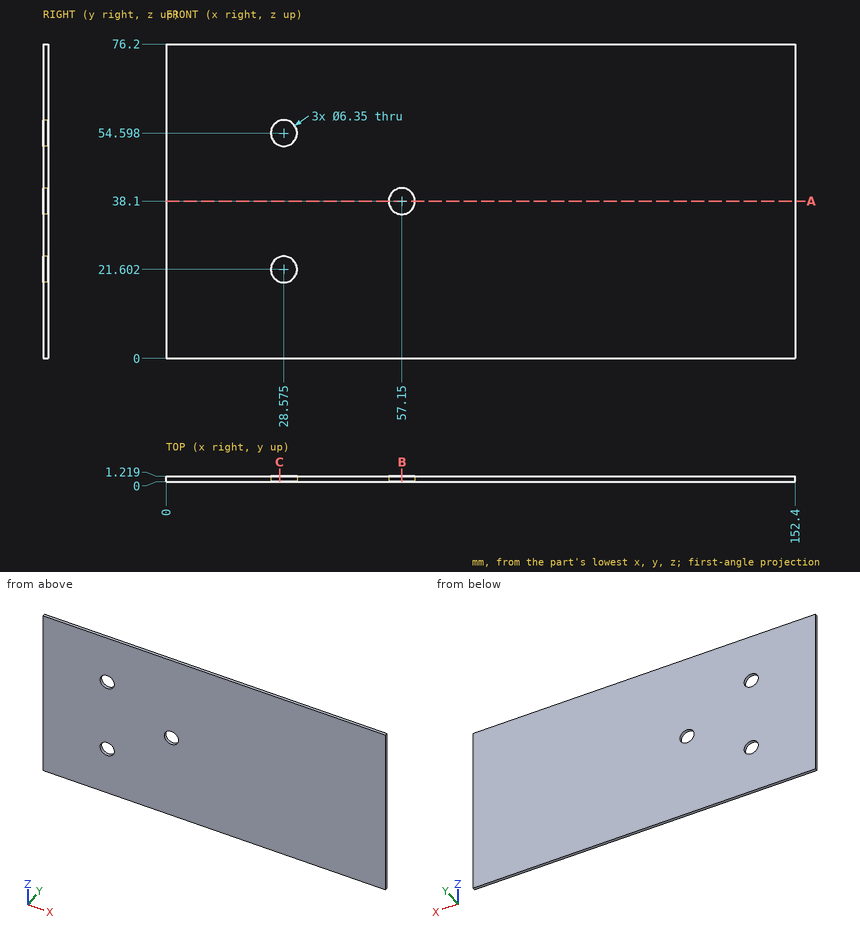
For this review, use the dimensioned drawing (mm, ordinates from the lowest corner) and the shaded views. Coordinates: 2 decimals unless noted, no trailing zeros. Loops run counter-clockwise (first coordinate to the right, second up) from the corner with the lowest first, then second, coordinate; pieces in that order, holes last. Notation, with made-up numbers: (4.25, 64.5) -> (41.25, 64.5) arc R17 cw to (41.25, 75.5) -> close; hole circle Ø11 at (74.5, -39.75). An arc over 180 degrees is marked (long way). Return JSON: item names as keys, results as strings. Group by question number.
(1) Consider section B-B, the plane x = 57.15. Give the boundary of the cut face in (y, z) (1 decimal).
(2) Consider section C-C, the plane x = 27.5. Give the boundary of the cut face in (y, z) (1 decimal).
(3) For pin 1 Ø5.5 at (x, z) = (57.15, 38.1) entering from -Y, flat-tipped, find the tip position at first contact; note if it passes through.
(4) Consider section A-A, the plane z = 38.1. Give the boundary of the cut face in (x, y) (1 decimal).
(5) To check wall thickness, follow L1, parallel to X at y = 0.95, z = 38; L2, parallel to X at y = 0.7, z = 22 (1 decimal); L3, parallel to Z at x = 55, y = 1. State the ranges of each line that lie inside material, in increasing order.
Results below:
{
 "1": {"outline": "(0, 0) -> (1.2, 0) -> (1.2, 34.9) -> (0, 34.9) -> close; (0, 41.3) -> (1.2, 41.3) -> (1.2, 76.2) -> (0, 76.2) -> close"},
 "2": {"outline": "(0, 0) -> (1.2, 0) -> (1.2, 18.6) -> (0, 18.6) -> close; (0, 24.6) -> (1.2, 24.6) -> (1.2, 51.6) -> (0, 51.6) -> close; (0, 57.6) -> (1.2, 57.6) -> (1.2, 76.2) -> (0, 76.2) -> close"},
 "3": {"pin 1": "passes through"},
 "4": {"outline": "(0, 0) -> (54, 0) -> (54, 1.2) -> (0, 1.2) -> close; (60.3, 0) -> (152.4, 0) -> (152.4, 1.2) -> (60.3, 1.2) -> close"},
 "5": {"L1": "x = 0 to 53.98, 60.32 to 152.4", "L2": "x = 0 to 25.4, 31.7 to 152.4", "L3": "z = 0 to 35.76, 40.44 to 76.2"}
}
